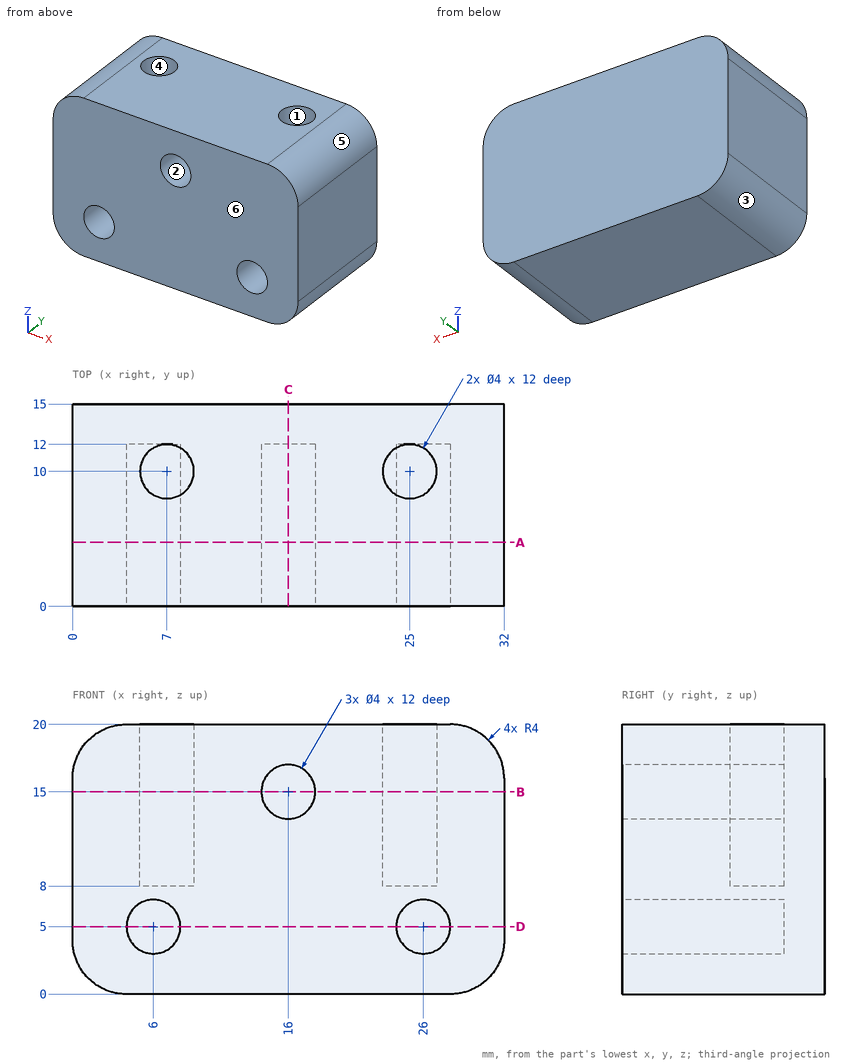
Here's the drawing with two shaded views (mm, measured from the low corner). I have some questions. A direction names the side the tool comes from. Round coordinates to 2 decimals unless told otherwise and drop trailing zeros. Loops run counter-clockwise (first coordinate to the right, second up) from the corner with the lowest first, then second, coordinate; pieces in that order, holes last. Notation, with made-up numbers: (32, 8) - (84, 8) arc R11 ccw to (84, 14) - close; hole circle Ø8 at (86, 3.5). An arc over 180 degrees is marked (long way). Use CSV: the item, a comma, the result in double quotes.
Item 1: Will these pins go through, and if not, where does the flat tip stop? pin 1 (3 mm diameter, centred on x = 6, z = 5, fed in from -Y); pin 2 (1.2 mm diameter, centred on x = 24, y = 10.5, fed in from +Z).
Here are the results:
pin 1,"stops at y = 12"
pin 2,"stops at z = 8"
Item 2: If we section it at A-A on y = 4.75: List the corners of the cut face in (x, z) for me, then the cut area to 3 significant figures.
Here are the results:
outline,"(0, 4) arc R4 ccw to (4, 0) - (28, 0) arc R4 ccw to (32, 4) - (32, 16) arc R4 ccw to (28, 20) - (4, 20) arc R4 ccw to (0, 16) - close; hole circle Ø4 at (6, 5); hole circle Ø4 at (16, 15); hole circle Ø4 at (26, 5)"
area,"589 mm²"
Item 3: If we section it at C-C on x = 16: List the corners of the cut face in (y, z) for me.
Here are the results:
outline,"(0, 0) - (15, 0) - (15, 20) - (0, 20) - (0, 17) - (12, 17) - (12, 13) - (0, 13) - close"
Item 4: If we mould it in two halves opening along Y, with no side actions, what happens to the marked faces 4, 5 and 6? For each: pulls with the +Y half, pulls with the -Y half, needs draft (parallel to the pull), parting line crosses it, or undercut.
Here are the results:
face 4,"undercut"
face 5,"needs draft"
face 6,"pulls with the -Y half"
Item 5: For the marked faces 1, 2 and 3, which set-ups out of +Z, -Z, +X, -X, +Y, -Y let a thin tool reach every point of the face, with its end or its side?
Here are the results:
face 1,"+Z"
face 2,"-Y"
face 3,"-Z, -X, +Y, -Y"
Item 6: If we section it at B-B on z = 15: List the corners of the cut face in (x, y) for me.
Here are the results:
outline,"(0, 0) - (14, 0) - (14, 12) - (18, 12) - (18, 0) - (32, 0) - (32, 15) - (0, 15) - close; hole circle Ø4 at (7, 10); hole circle Ø4 at (25, 10)"
Item 7: I need wall thicknesses on L1, parallel to X at y = 9.25, z = 5; L2, parallel to Y at x = 25, z = 16.5; L3, parallel to X at y = 7.5, z = 13.25. Which ranges of each line are inside material? Lowest first, please. Write a range as [from, to].
Here are the results:
L1,"x = [0, 4], [8, 24], [28, 32]"
L2,"y = [0, 8], [12, 15]"
L3,"x = [0, 15.03], [16.97, 32]"
Item 8: If we section it at D-D on z = 5: List the corners of the cut face in (x, y) for me.
Here are the results:
outline,"(0, 0) - (4, 0) - (4, 12) - (8, 12) - (8, 0) - (24, 0) - (24, 12) - (28, 12) - (28, 0) - (32, 0) - (32, 15) - (0, 15) - close"
